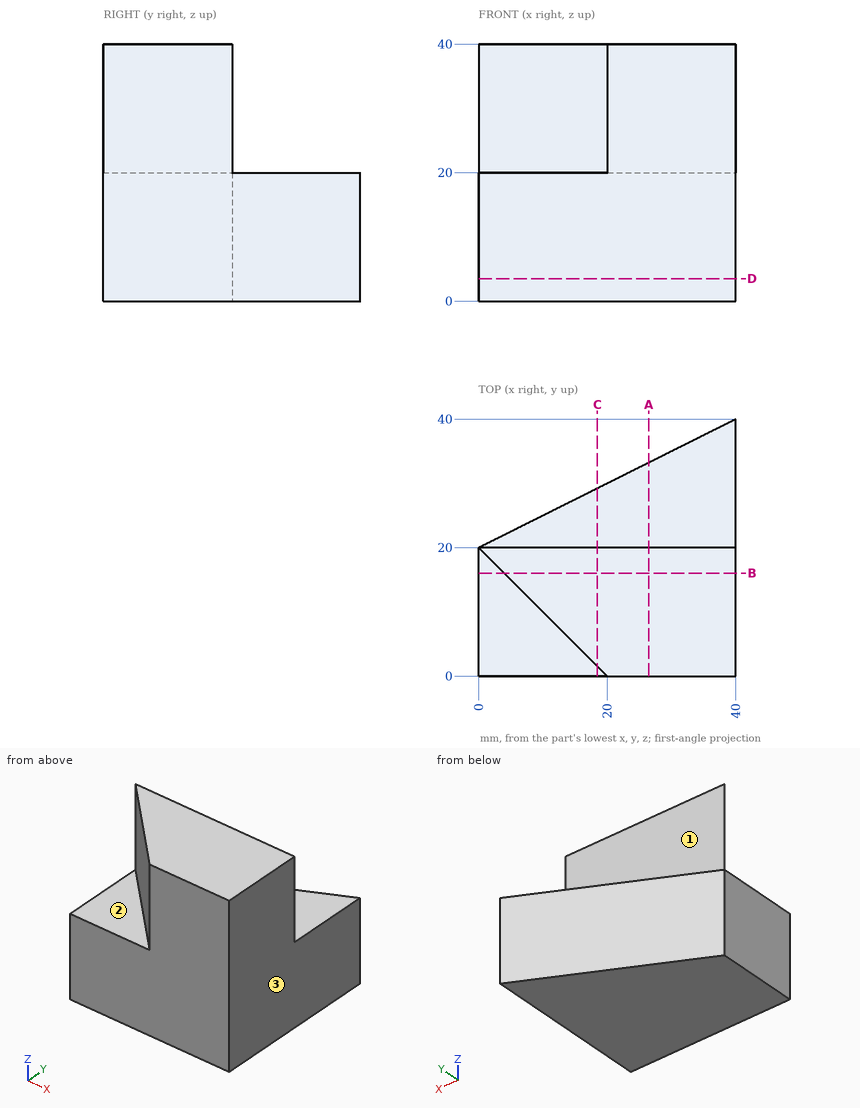
Source: three-view drawing plus pictorial views. Frame: mm from the lowest corner of the part. A direction names the side the tool comes from. Give positions to 0.01 mm unless a question says otherwise; leave off trailing zeros. Order: outer loops, then holes, each group sorted by start corner. A loop starts at its lowest first (then second) coordinate and runs counter-clockwise, first axis right, second up. Notation, with made-up numbers: (37.25, 35.25) -> (69.25, 35.25) arc R36 cw to (69.25, 74.25) -> close; hole circle Ø10 at (62, -10). An arc over 180 degrees is marked (long way). Put each result on its own line as item: value.
Q1. Section D-D, the plane z = 3.5. Return loops of the section in (x, y).
Here are the results:
outline: (0, 0) -> (40, 0) -> (40, 40) -> (0, 20) -> close
Q2. Pin query (flat end, axial travel): pin 1 (3 mm diameter, centred on x = 12.5, y = 22, fed in from +Z); pin 2 (6 mm diameter, centred on x = 17.5, z = 30.5, fed in from +Y). Return the tip coordinate at first contact, or that it passes through.
Here are the results:
pin 1: stops at z = 20
pin 2: stops at y = 20
Q3. Section B-B, the plane y = 16. Return loops of the section in (x, z).
Here are the results:
outline: (0, 0) -> (40, 0) -> (40, 40) -> (4, 40) -> (4, 20) -> (0, 20) -> close
Q4. Section A-A, the plane x = 26.5. Return loops of the section in (y, z), then the cut area to 4 significant figures.
Here are the results:
outline: (0, 0) -> (33.25, 0) -> (33.25, 20) -> (20, 20) -> (20, 40) -> (0, 40) -> close
area: 1,065 mm^2
Q5. Reachability of the marked faces 1, 2 and 3 from +Z, -Z, +X, -X, +Y, -Y: full face, straight path, thin tool, end or side. Return the list, or none.
Here are the results:
face 1: +Z, +X, -X, +Y
face 2: +Z, -X, -Y
face 3: +Z, -Z, +X, +Y, -Y
Q6. Material intervals for L1, parallel to Z at x = 34, y = 23.5; L2, parallel to Y at x = 38, z = 10.5, sorted ascending.
Here are the results:
L1: z = 0 to 20
L2: y = 0 to 39
Q7. Section C-C, the plane x = 18.5. Return loops of the section in (y, z).
Here are the results:
outline: (0, 0) -> (29.25, 0) -> (29.25, 20) -> (20, 20) -> (20, 40) -> (1.5, 40) -> (1.5, 20) -> (0, 20) -> close
